Input: dimensioned drawing with shaded views. Units: mm. Origin: part minimum x, y, z. Round coordinates to 2 decimals unless told otherwise and drop trailing zeros. Loops run counter-clockwise (first coordinate to the right, second up) from the corner with the lowest first, then second, coordinate; pieces in that order, holes last. Notation, with made-up numbers: (33, 1.5) -> (76, 1.5) arc R15 ccw to (76, 23.5) -> close; hole circle Ø10 at (29.25, 11). An arc over 180 degrees is marked (long way). Answer as a JSON object with one key per item and string values.
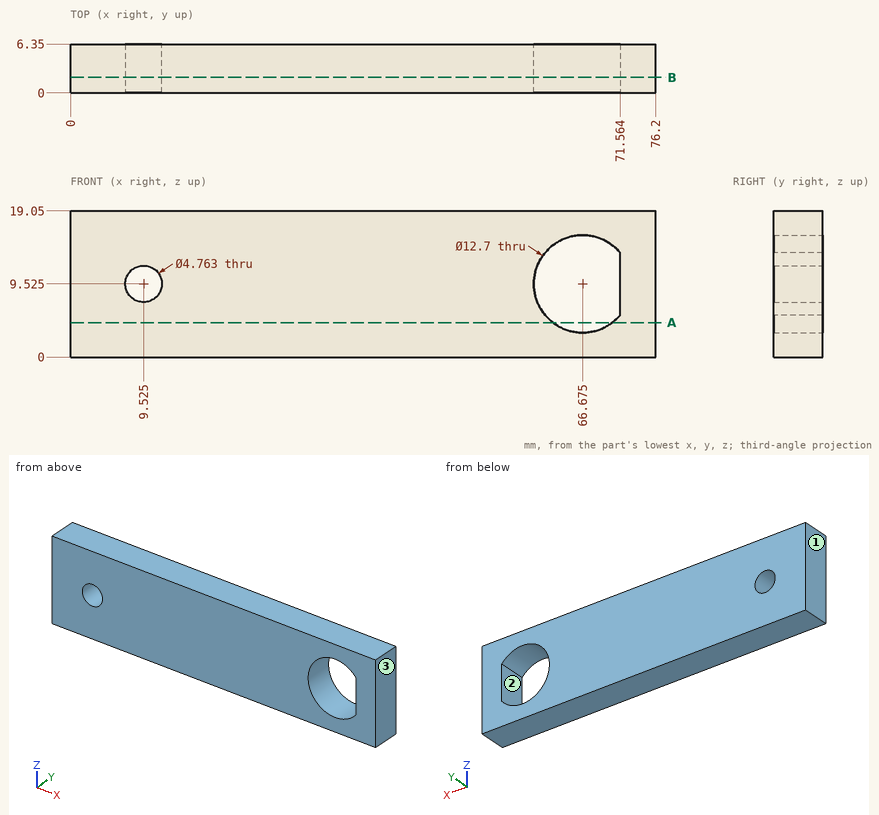
1) Draft query along X for the marked faces 1, 2 and 3. Return one class per face: +X half, -X half, draft (parallel to the pull), parting line (faces both ways), or undercut.
Output:
{"face 1": "-X half", "face 2": "undercut", "face 3": "+X half"}
2) Ray query, probe 1 along X at (y, z) = (2.5, 10) (1 decimal); probe 2 along X at (y, z) = (5.5, 8.25) (1 decimal); probe 3 along X at (y, z) = (1, 14). Return the intervals inside material, ascending.
Output:
{"probe 1": "x = 0 to 7.2, 11.9 to 60.3, 71.6 to 76.2", "probe 2": "x = 0 to 7.5, 11.5 to 60.5, 71.6 to 76.2", "probe 3": "x = 0 to 62.17, 71.18 to 76.2"}
3) Section A-A, the plane z = 4.5. Output: boundary loops of the cut face in (x, y).
Output:
{"outline": "(0, 0) -> (62.79, 0) -> (62.79, 6.35) -> (0, 6.35) -> close; (70.56, 0) -> (76.2, 0) -> (76.2, 6.35) -> (70.56, 6.35) -> close"}
4) Section B-B, the plane y = 2. Count the separate pieces of the cut face and the enclosed holes in it, plus the area to 4 significant figures.
Output:
{"separate pieces": "1", "enclosed holes": "2", "area": "1,315 mm^2"}
